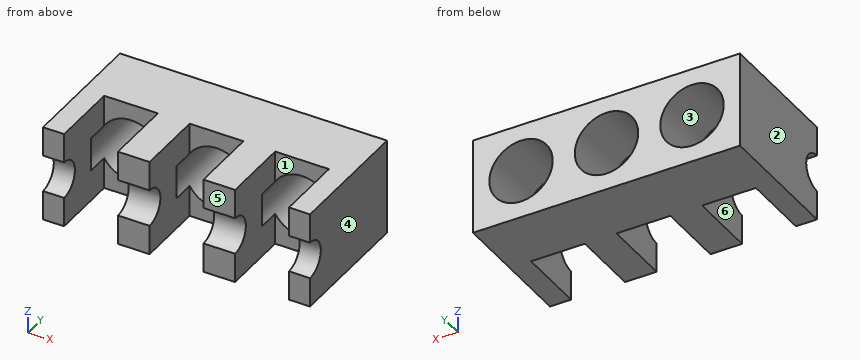
```python
from build123d import *

# Parameters (mm, degrees)
SKETCH1_W           = 253
SKETCH1_H           = 91
BOSS_EXTRUDE1_DEPTH = 125
SKETCH2_W           = 51
SKETCH2_H           = 65
CUT_EXTRUDE1_DEPTH  = 92
SKETCH3_R           = 30.05
CUT_EXTRUDE2_DEPTH  = 81
SKETCH4_R           = 17.5
CUT_EXTRUDE3_DEPTH  = 254


with BuildPart() as part:
    # Sketch1 → Boss-Extrude1 (new body)
    with BuildSketch(Plane(origin=(0, 0, 0), x_dir=(1, 0, 0), z_dir=(0, 1, 0))):
        with Locations((126.5, -45.5)):
            Rectangle(SKETCH1_W, SKETCH1_H)
    extrude(amount=BOSS_EXTRUDE1_DEPTH)

    # Sketch2 → Cut-Extrude1 (cut, through all)
    with BuildSketch(Plane.XY.offset(91)):
        with Locations((45.5, 32.5)):
            Rectangle(SKETCH2_W, SKETCH2_H)
        with Locations((126.5, 32.5)):
            Rectangle(SKETCH2_W, SKETCH2_H)
        with Locations((207.5, 32.5)):
            Rectangle(SKETCH2_W, SKETCH2_H)
    extrude(amount=-CUT_EXTRUDE1_DEPTH, mode=Mode.SUBTRACT)

    # Sketch3 → Cut-Extrude2 (cut)
    with BuildSketch(Plane(origin=(0, 125, 0), x_dir=(1, 0, 0), z_dir=(0, 1, 0))):
        with Locations((45.5, -45.5)):
            Circle(SKETCH3_R)
        with Locations((126.5, -45.5)):
            Circle(SKETCH3_R)
        with Locations((207.5, -45.5)):
            Circle(SKETCH3_R)
    extrude(amount=-CUT_EXTRUDE2_DEPTH, mode=Mode.SUBTRACT)

    # Sketch4 → Cut-Extrude3 (cut, through all)
    with BuildSketch(Plane(origin=(253, 0, 0), x_dir=(0, 0, -1), z_dir=(1, 0, 0))):
        with Locations((-45.5, 0)):
            Circle(SKETCH4_R)
    extrude(amount=-CUT_EXTRUDE3_DEPTH, mode=Mode.SUBTRACT)


solid = part.part
```
Geometry check sheet. Reference: the model listing, model coordinates, mm. Face numbers are marked on the shaded views. A direction names the side the tool comes from. Coordinates: 2 decimals unless noted, no trailing zeros. Write each loop counter-clockwise with the first axis right and the second up, starting at its lowest first coordinate (ties: lowest second). Pieces come first, ordered by that corner, then holes. Notation, with made-up numbers: M 23,70.25 L 63,70.25 A10 ccw 63,82.25 Z; hole C -8.5,55 d6. An arc over 180 degrees is marked long. Use one line per item in the form item = value. Start each with the question number.
1) Thickness scan on probe 1 along X at (y, z) = (18.5, 82); probe 2 along X at (y, z) = (102, 45.5); probe 3 along Z at (x, y) = (101, 85). Record the ranges inside material, lowest first. Write a range as from..to.
2) Set-up check for the marked faces 1, 2 and 3: record each of +Z, -Z, +X, -X, +Y, -Y from which the full face is reachable in a straight line by a thin tool's end or side.
3) Section check B-B on z = 45.5. Enter the section's corners in (x, y), and give its area (3 significant figures).
4) Section check C-C on x = 126.5. Enter the section's corners in (y, z), and give its area (3 significant figures).
5) Section check D-D on y = 72. Enter the section's corners in (x, z), and give its area (3 significant figures).
6) Section check A-A on y = 38. Enter the section's corners in (x, z).
7) Release check for a two-part mould opening along X. For the marked faces 4, 5 and 6 record: pulls with the +X half, pulls with the -X half, needs draft (parallel to the pull), parting line crosses it, or undercut.
8) Go/stop test with flat-tipped pins: pin 1 Ø5 at (x, z) = (236, 42.5) entering from +Y; pin 2 Ø1.4 at (x, z) = (154, 38.5) entering from +Y; pin 3 Ø9 at (x, z) = (123, 18.5) entering from -Y. Record where each tip stops, or that it passes through.
Responses:
q1.probe_1 = 0..20, 71..101, 152..182, 233..253
q1.probe_2 = 0..15.45, 75.55..96.45, 156.55..177.45, 237.55..253
q1.probe_3 = 0..29.6, 61.4..91
q2.face_1 = +Z, -Z, -Y
q2.face_2 = +Z, -Z, -X, +Y, -Y
q2.face_3 = +Y
q3.outline = M 0,17.5 L 20,17.5 L 20,44 L 15.45,44 L 15.45,125 L 0,125 Z; M 71,17.5 L 101,17.5 L 101,44 L 96.45,44 L 96.45,125 L 75.55,125 L 75.55,44 L 71,44 Z; M 152,17.5 L 182,17.5 L 182,44 L 177.45,44 L 177.45,125 L 156.55,125 L 156.55,44 L 152,44 Z; M 233,17.5 L 253,17.5 L 253,125 L 237.55,125 L 237.55,44 L 233,44 Z
q3.area = 8,540 mm2
q4.outline = M 65,0 L 125,0 L 125,15.45 L 65,15.45 Z; M 65,75.55 L 125,75.55 L 125,91 L 65,91 Z
q4.area = 1,850 mm2
q5.outline = M 0,0 L 253,0 L 253,91 L 0,91 Z; hole C 45.5,45.5 d60.1; hole C 126.5,45.5 d60.1; hole C 207.5,45.5 d60.1
q5.area = 14,500 mm2
q6.outline = M 0,0 L 20,0 L 20,91 L 0,91 Z; M 71,0 L 101,0 L 101,91 L 71,91 Z; M 152,0 L 182,0 L 182,91 L 152,91 Z; M 233,0 L 253,0 L 253,91 L 233,91 Z
q7.face_4 = pulls with the +X half
q7.face_5 = needs draft
q7.face_6 = undercut
q8.pin_1 = 125
q8.pin_2 = 44
q8.pin_3 = 65
